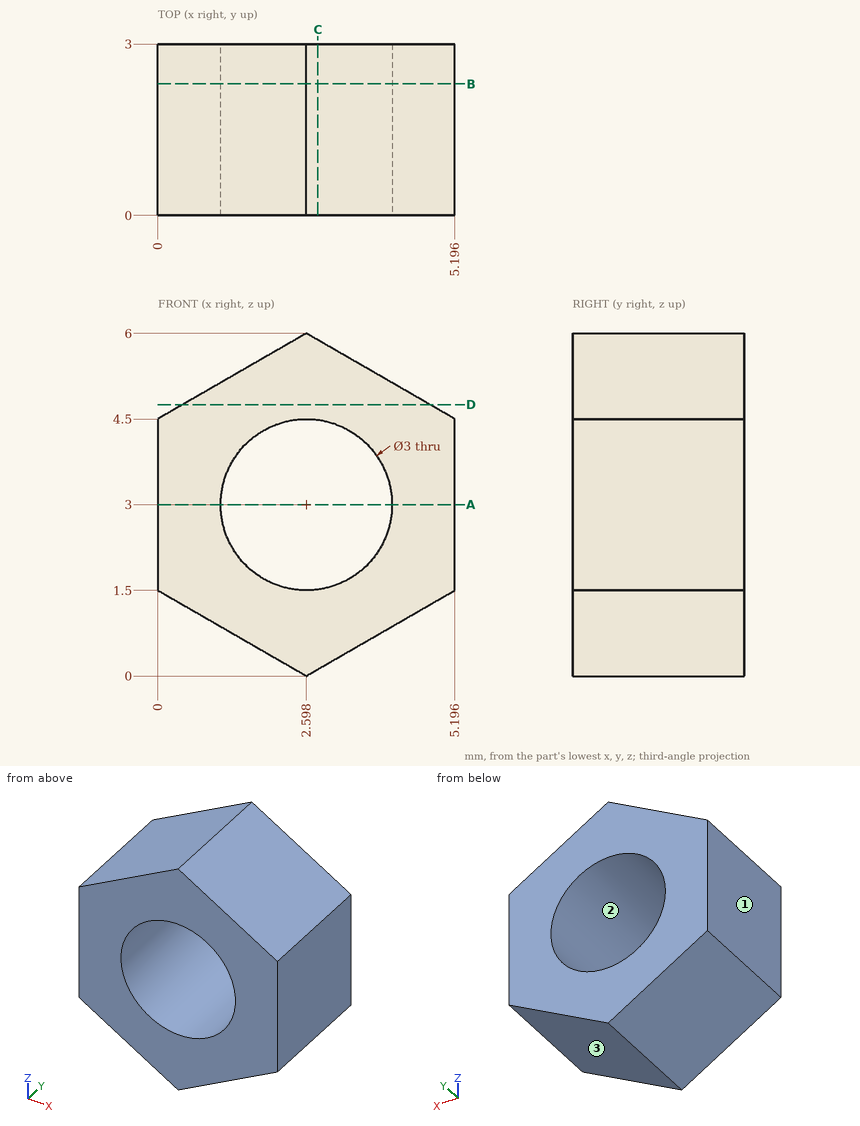
Design review of the part shown in the three views and the two pictorial views. Dimensions are in mm from the part's minimum x, y and z. Round coordinates to 2 decimals unless told otherwise and drop trailing zeros. Write each loop counter-clockwise with the first axis right and the second up, starting at its lowest first coordinate (ties: lowest second). Pieces come first, ordered by that corner, then holes. Notation, with made-up numbers: (41.5, 56.25) -> (68.5, 56.25) arc R11 cw to (68.5, 74.25) -> close; hole circle Ø3 at (87, 84). An arc over 180 degrees is marked (long way). Answer as a JSON object with one key per item and string values.
1. We need section C-C on x = 2.8. State the section outline as (y, z) points.
Results found:
{"outline": "(0, 0.12) -> (3, 0.12) -> (3, 1.51) -> (0, 1.51) -> close; (0, 4.49) -> (3, 4.49) -> (3, 5.88) -> (0, 5.88) -> close"}
2. We need section B-B on y = 2.3. State the section outline as (x, z) points, and give its area (3 significant figures).
Results found:
{"outline": "(0, 1.5) -> (2.6, 0) -> (5.2, 1.5) -> (5.2, 4.5) -> (2.6, 6) -> (0, 4.5) -> close; hole circle Ø3 at (2.6, 3)", "area": "16.3 mm^2"}
3. The part is to be moulded in two halves that separate along X. For the marked faces 1, 2 and 3, say which applies: pulls with the +X half, pulls with the -X half, needs draft (parallel to the pull), parting line crosses it, or undercut.
Results found:
{"face 1": "pulls with the -X half", "face 2": "undercut", "face 3": "pulls with the +X half"}
4. We need section A-A on z = 3. State the section outline as (x, y) points.
Results found:
{"outline": "(0, 0) -> (1.1, 0) -> (1.1, 3) -> (0, 3) -> close; (4.1, 0) -> (5.2, 0) -> (5.2, 3) -> (4.1, 3) -> close"}
5. We need section D-D on z = 4.75. State the section outline as (x, y) points.
Results found:
{"outline": "(0.43, 0) -> (4.76, 0) -> (4.76, 3) -> (0.43, 3) -> close"}
6. Clearance check with flat-ended pins moving along their axes: pin 1 (1 mm diameter, centred on x = 1, y = 0.5, fed in from -Z); pin 2 (1.8 mm diameter, centred on x = 2.6, z = 3, fed in from -Y). State where each tip first meets the part, or that it passes through.
Results found:
{"pin 1": "stops at z = 0.63", "pin 2": "passes through"}
7. To check wall thickness, follow line 1 along Z through (x, y) = (1.65, 1.65); line 2 along X through (y, z) = (0.4, 3.2) (1 decimal); line 3 along X through (y, z) = (2.7, 4.15) (1 decimal). State the ranges of each line that lie inside material, in increasing order.
Results found:
{"line 1": "z = 0.55 to 1.84, 4.16 to 5.45", "line 2": "x = 0 to 1.1, 4.1 to 5.2", "line 3": "x = 0 to 1.6, 3.6 to 5.2"}
